The listing builds one solid part. Answer for the finished solid, in the listing's coordinates (mm). Face numbers are marked on the shaded views. A direction names the side the tool comes from. Round coordinates to 2 decimals unless told otherwise and drop trailing zeros. Write each loop counter-clockwise with the first axis right and the second up, starting at its lowest first coordinate (ties: lowest second). Pieces come first, ordered by that corner, then holes. Notation, with made-up numbers: M -15.75,88 L 9.25,88 A13 cw 9.25,104 Z; hole C 21,-28 d10. An arc over 180 degrees is marked long. Put each result on its own line as item: value. Start each with the question number.
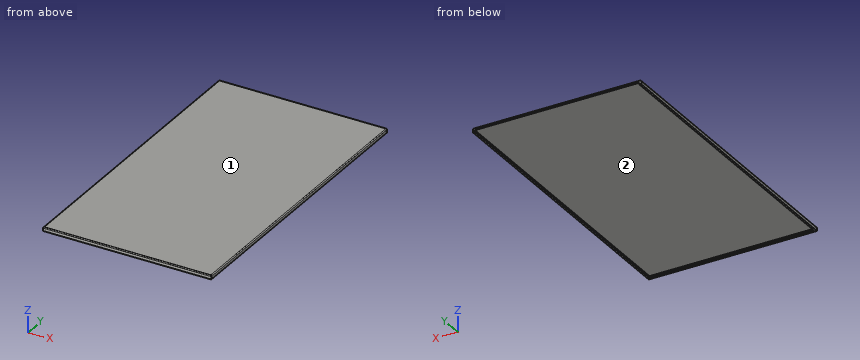
```python
from build123d import *

# Parameters (mm, degrees)
F0_W     = 1143
F0_H     = 2032
F1_DEPTH = 25.4
F2_T     = -12.7
F3_R     = 6.35


with BuildPart() as f1:
    # F0 (on Top) → F1 (new body)
    with BuildSketch(Plane.XY):
        with Locations((571.5, 1016)):
            Rectangle(F0_W, F0_H)
    extrude(amount=F1_DEPTH)

    # F2
    f2_openings = [f1.faces().sort_by_distance(p)[0] for p in [
        (571.5, 1016, 0),
        (571.5, 2032, 12.7),
    ]]
    offset(amount=F2_T, openings=f2_openings)

    # F3
    f3_edges = [f1.edges().sort_by_distance(p)[0] for p in [
        (1143, 1016, 25.4),
        (571.5, 0, 25.4),
        (0, 1016, 25.4),
    ]]
    fillet(f3_edges, radius=F3_R)


solid = f1.part
```
Item 1: Section A-A (y = 1180) is taken. Give the vertices of the cut face in (x, z).
Item 2: Flat-ended cylindrical pins translate along their axes: pin 1 (4 mm diameter, centred on x = 497.5, y = 1417.5, fed in from -Z); pin 2 (10 mm diameter, centred on x = 515.5, z = 7.5, fed in from +Y). Find the tip coordinate at first contact, or state that the pin passes through.
Item 3: Section C-C (z = 5) is taken. Give the vertices of the cut face in (x, y).
Item 4: Consider line 1 along X through (y, z) = (455, 3.75); line 2 along Z through (x, y) = (539, 1772); line 3 along Y through (x, z) = (290, 5.75). Determine where each line is inside the solid, lowest interval first. Write a range as [from, to].
Item 5: Section B-B (x = 843.5) is taken. Give the vertices of the cut face in (y, z), and give its area (3 significant figures).
Item 6: Which of the six approach directions +Z, -Z, +X, -X, +Y, -Y give full straight-line access (tool end or side, diameter ignored) to the marked faces 1 and 2?
Output values:
1. outline: M 0,0 L 12.7,0 L 12.7,12.7 L 1130.3,12.7 L 1130.3,0 L 1143,0 L 1143,19.05 A6.35 ccw 1136.65,25.4 L 6.35,25.4 A6.35 ccw 0,19.05 Z
2. pin 1: stops at z = 12.7
2. pin 2: stops at y = 12.7
3. outline: M 0,0 L 1143,0 L 1143,2032 L 1130.3,2032 L 1130.3,12.7 L 12.7,12.7 L 12.7,2032 L 0,2032 Z
4. line 1: x = [0, 12.7], [1130.3, 1143]
4. line 2: z = [12.7, 25.4]
4. line 3: y = [0, 12.7]
5. outline: M 0,0 L 12.7,0 L 12.7,12.7 L 2032,12.7 L 2032,25.4 L 6.35,25.4 A6.35 ccw 0,19.05 Z
5. area: 26,000 mm^2
6. face 1: +Z, +X, -X, +Y, -Y
6. face 2: -Z, +Y
